For this review, use the dimensioned drawing (mm, ordinates from the lowest corner) and the shaded views. A direction names the side the tool comes from. Give positions to 0.01 mm unless a question says otherwise; leave off trailing zeros. Order: outer loops, then holes, each group sorted by start corner. A loop starts at its lowest first (then second) coordinate and runs counter-clockwise, first axis right, second up. Notation, with made-up numbers: M 69.5,65 L 76.5,65 A30 cw 76.5,94 Z; hole C 64,72.25 d7. An arc over 180 degrees is marked long. Use CSV: the item, a comma, the result in double quotes. Start each with the question number.
(1) Consider section D-D (y = 8.25). Write out the cut boundary in (x, z), and give its area (3 significant figures).
(2) Consider section C-C (y = 20.25). Write out the cut boundary in (x, z).
(3) Consider section B-B (x = 2.3). Write out the cut boundary in (y, z).
(4) Wall thickness on L1, parallel to X at y = 18.5, z = 3.4: over which ranges is the line inside the solid? List them lowest first. Write a range as from..to.
(5) Consider section A-A (z = 1.2). Write out the cut boundary in (x, y).
(6) Draft analysis for pull direction Z (two halves, no side actions). For the marked faces 3, 4 and 5, state which applies: pulls with the +Z half, pulls with the -Z half, needs draft (parallel to the pull), parting line crosses it, or undercut.
(7) Tool access review of the marked faces 1 and 2: name each direction out of +Z, -Z, +X, -X, +Y, -Y from which nothing blocks a thin tool from reaching the whole face with its end or side.
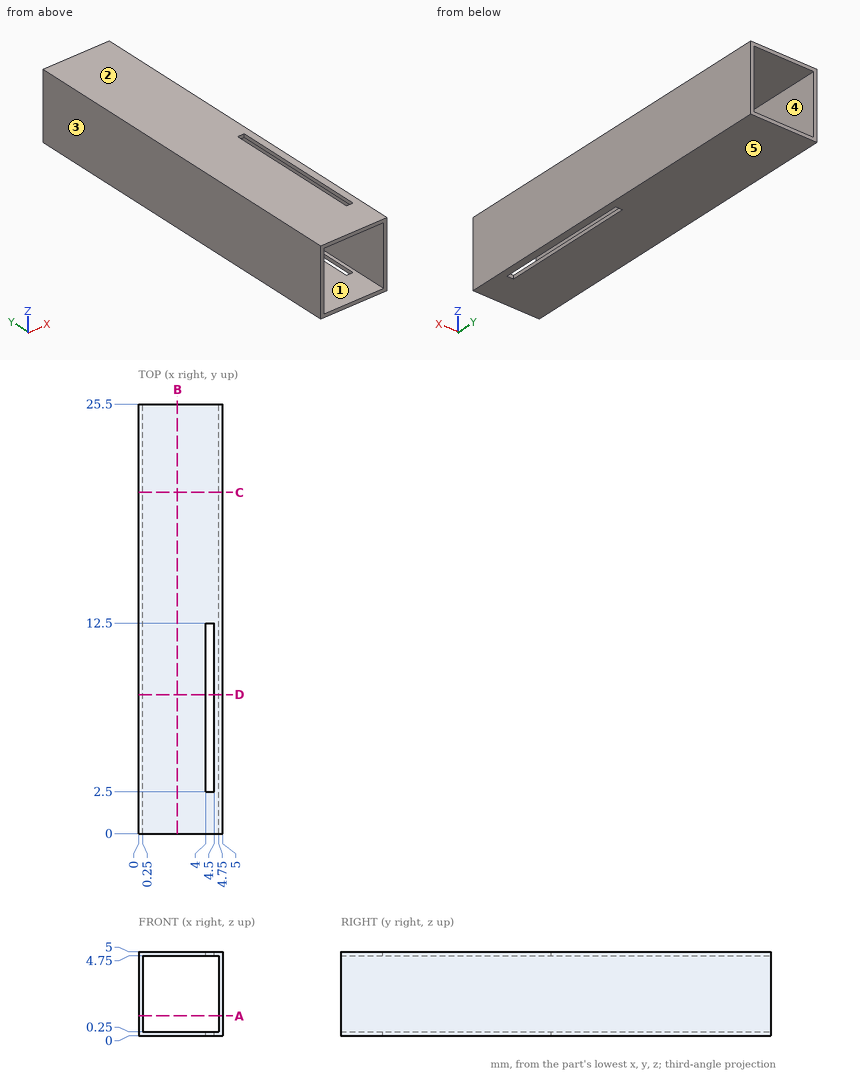
Check result:
1,outline,"M 0,0 L 4,0 L 4,0.25 L 0.25,0.25 L 0.25,4.75 L 4,4.75 L 4,5 L 0,5 Z; M 4.5,0 L 5,0 L 5,5 L 4.5,5 L 4.5,4.75 L 4.75,4.75 L 4.75,0.25 L 4.5,0.25 Z"
1,area,"4.50 mm^2"
2,outline,"M 0,0 L 5,0 L 5,5 L 0,5 Z; hole M 0.25,0.25 L 4.75,0.25 L 4.75,4.75 L 0.25,4.75 Z"
3,outline,"M 0,0 L 25.5,0 L 25.5,0.25 L 0,0.25 Z; M 0,4.75 L 25.5,4.75 L 25.5,5 L 0,5 Z"
4,L1,"x = 0..0.25, 4.75..5"
5,outline,"M 0,0 L 0.25,0 L 0.25,25.5 L 0,25.5 Z; M 4.75,0 L 5,0 L 5,25.5 L 4.75,25.5 Z"
6,face 3,"needs draft"
6,face 4,"undercut"
6,face 5,"pulls with the -Z half"
7,face 1,"+Y, -Y"
7,face 2,"+Z, +X, -X, +Y, -Y"
